Source: three-view drawing plus pictorial views. Frame: mm from the lowest corner of the part. A direction names the side the tool comes from. Give positions to 0.01 mm unless a question says otherwise; leave off trailing zeros. Loops run counter-clockwise (first coordinate to the right, second up) from the corner with the lowest first, then second, coordinate; pieces in that order, holes last. Notation, with made-up numbers: M -29,75 L 6,75 A16 ccw 6,101 Z; hole C -8,-5.75 d6. An arc over 180 degrees is marked long. Write item = value, one per line.
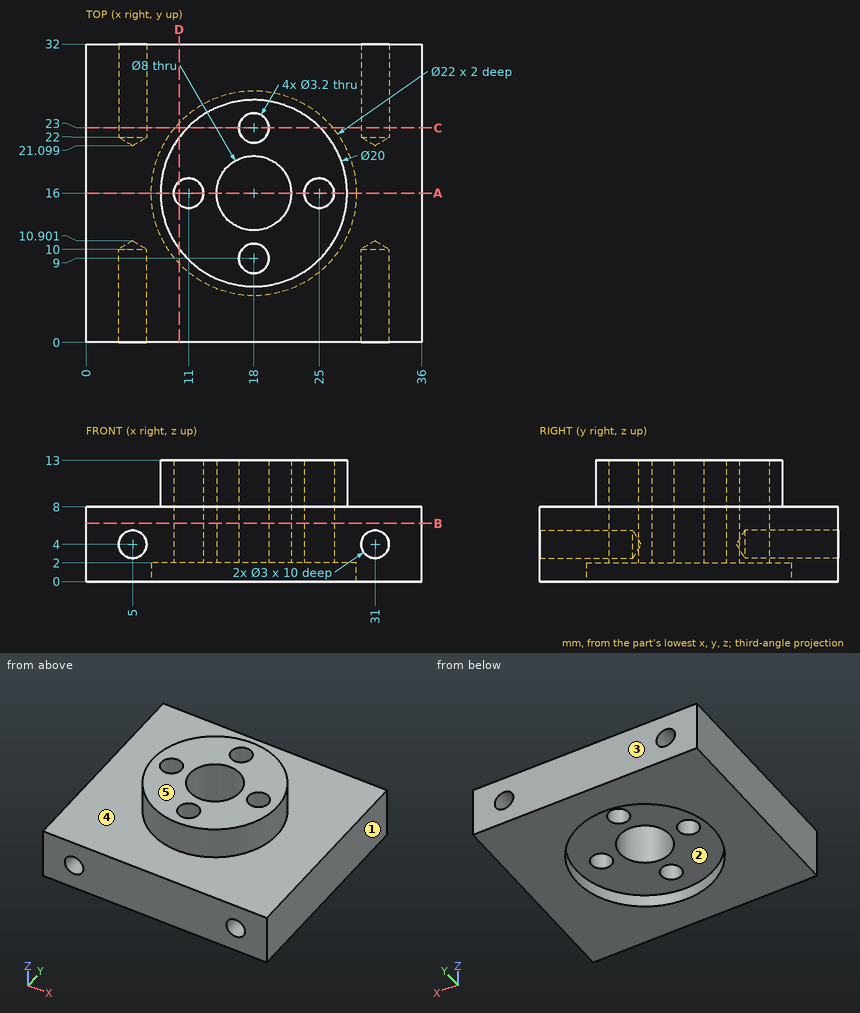
1. Cut plane C-C, the plane y = 23. Return the cut outline in (x, z) (1 decimal), then the cut area to 3 significant figures.
Derived:
outline = M 0,0 L 9.5,0 L 9.5,2 L 16.4,2 L 16.4,13 L 10.9,13 L 10.9,8 L 0,8 Z; M 19.6,2 L 26.5,2 L 26.5,0 L 36,0 L 36,8 L 25.1,8 L 25.1,13 L 19.6,13 Z; hole C 5,4 d3; hole C 31,4 d3
area = 276 mm²
2. Material intervals for probe 1 along X at (y, z) = (16, 8.25); probe 2 along Y at (x, z) = (18, 9); probe 3 along Z at (x, y) = (5, 6), sorted ascending. Write a range as from..to.
Derived:
probe_1 = 8..9.4, 12.6..14, 22..23.4, 26.6..28
probe_2 = 6..7.4, 10.6..12, 20..21.4, 24.6..26
probe_3 = 0..2.5, 5.5..8
3. Cut plane A-A, the plane y = 16. Return the cut outline in (x, z).
Derived:
outline = M 0,0 L 7,0 L 7,2 L 9.4,2 L 9.4,13 L 8,13 L 8,8 L 0,8 Z; M 12.6,2 L 14,2 L 14,13 L 12.6,13 Z; M 22,2 L 23.4,2 L 23.4,13 L 22,13 Z; M 26.6,2 L 29,2 L 29,0 L 36,0 L 36,8 L 28,8 L 28,13 L 26.6,13 Z
4. Pull-direction query (Y, two-part tool) for the marked faces 1, 2 and 3; classes: +Y half, -Y half, draft (parallel to the pull), parting line (faces both ways), or undercut.
Derived:
face_1 = draft
face_2 = undercut
face_3 = +Y half
5. Cut plane D-D, the plane x = 10. Return the cut outline in (y, z), then the cut area to 3 significant figures.
Derived:
outline = M 0,0 L 8.45,0 L 8.45,2 L 14.75,2 L 14.75,13 L 10,13 L 10,8 L 0,8 Z; M 17.25,2 L 23.55,2 L 23.55,0 L 32,0 L 32,8 L 22,8 L 22,13 L 17.25,13 Z
area = 258 mm²
6. First-contact query: pin 1 Ø4 at (x, y) = (25, 16) entering from +Z; pin 2 Ø1.5 at (x, y) = (19, 9.5) entering from -Z. Flat tips, straight axial feed; report the tip coordinate or a pass-through.
Derived:
pin_1 = 13
pin_2 = 2
7. Cut plane B-B, the plane z = 6.25. Return the cut outline in (x, y).
Derived:
outline = M 0,0 L 36,0 L 36,32 L 0,32 Z; hole C 11,16 d3.2; hole C 18,16 d8; hole C 18,9 d3.2; hole C 18,23 d3.2; hole C 25,16 d3.2
8. Reachability of the marked faces 4 and 5 from +Z, -Z, +X, -X, +Y, -Y: full face, straight path, thin tool, end or side. Return the list, or none.
Derived:
face_4 = +Z
face_5 = +Z, +X, -X, +Y, -Y
